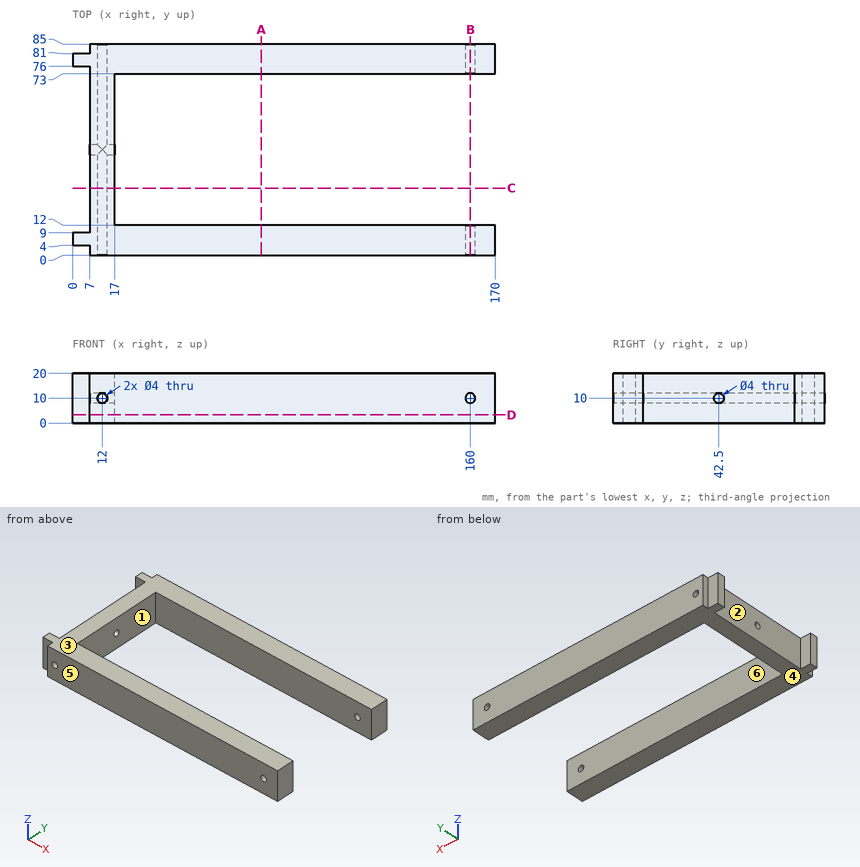
Verification items for this drawing (mm, ordinates from the low corner). A direction names the side the tool comes from. Coordinates: 2 decimals unless noted, no trailing zeros. Write each loop counter-clockwise with the first axis right and the second up, starting at its lowest first coordinate (ties: lowest second). Pieces come first, ordered by that corner, then holes. Notation, with made-up numbers: M 16,11 L 56,11 A23 cw 56,42 Z; hole C 1.25,1.25 d2. An arc over 180 degrees is marked long. Use one line per item in the form item = value. Start each with the question number.
1) Go/stop test with flat-tipped pins: pin 1 Ø6.5 at (x, z) = (12, 10) entering from -Y; pin 2 Ø3.5 at (x, z) = (5, 10.5) entering from -Y; pin 3 Ø1 at (y, z) = (26.5, 12.5) entering from +X; pin 4 Ø3 at (y, z) = (1.5, 7) entering from -X. Record where each tip stops, or that it passes through.
2) Section check C-C on y = 27. Enter the section's corners in (x, z).
3) Thickness scan on probe 1 along Y at (x, z) = (87, 9.5); probe 2 along Z at (x, y) = (12, 31); probe 3 along X at (y, z) = (59, 10). Record the ranges inside material, lowest first. Write a range as from..to.
4) Section check A-A on x = 76. Enter the section's corners in (y, z).
5) Section check D-D on z = 3.25. Enter the section's corners in (x, y).
6) Release check for a two-part mould opening along Y. For the marked faces 4, 5 and 6 record: pulls with the +Y half, pulls with the -Y half, needs draft (parallel to the pull), parting line crosses it, or undercut.
7) Section check B-B on x = 160. Enter the section's corners in (y, z).
8) Set-up check for the marked faces 1, 2 and 3: record each of +Z, -Z, +X, -X, +Y, -Y from which the full face is reachable in a straight line by a thin tool's end or side.
Responses:
q1.pin_1 = 0
q1.pin_2 = 4
q1.pin_3 = 17
q1.pin_4 = 7
q2.outline = M 7,0 L 17,0 L 17,20 L 7,20 Z; hole C 12,10 d4
q3.probe_1 = 0..12, 73..85
q3.probe_2 = 0..8, 12..20
q3.probe_3 = 7..10, 14..17
q4.outline = M 0,0 L 12,0 L 12,20 L 0,20 Z; M 73,0 L 85,0 L 85,20 L 73,20 Z
q5.outline = M 0,4 L 7,4 L 7,0 L 170,0 L 170,12 L 17,12 L 17,73 L 170,73 L 170,85 L 7,85 L 7,81 L 0,81 L 0,76 L 7,76 L 7,9 L 0,9 Z
q6.face_4 = needs draft
q6.face_5 = pulls with the -Y half
q6.face_6 = undercut
q7.outline = M 0,0 L 12,0 L 12,8 L 0,8 Z; M 0,12 L 12,12 L 12,20 L 0,20 Z; M 73,0 L 85,0 L 85,8 L 73,8 Z; M 73,12 L 85,12 L 85,20 L 73,20 Z
q8.face_1 = +Z, -Z, +X
q8.face_2 = +Z, -Z, -X
q8.face_3 = +Z, +X, -X, +Y, -Y
